For this review, take the finished solid that the model builds, in its own axes (mm). Face numbers are marked on the shaded views. A direction names the side the tool comes from. Coordinates: 2 decimals unless noted, no trailing zeros. Order: outer loops, then holes, each group sorted by start corner. A loop starts at its lowest first (then second) coordinate and runs counter-clockwise, first axis right, second up. Notation, with made-up numbers: (28, 37.5) -> (65, 37.5) arc R37 cw to (65, 73.5) -> close; hole circle Ø8 at (57, 47.25). An arc over 180 degrees is marked (long way). Answer as a JSON object with one key per item and string values. Group by question number.
1) Add section B-B, the plane z = 1.75. Write out the cut boundary in (x, y), then the cut area to 3 significant figures.
2) For pin 1 (4 mm diameter, centred on x = -3, z = 0, fed in from +Y); pin 2 (4 mm diameter, centred on x = -2.5, z = 3, fed in from +Y); pin 3 (6.5 mm diameter, centred on y = -21, z = 4, fed in from +X), all flat-tipped, find the tip position at first contact; note any pin that passes through.
3) Wall thickness on L1, parallel to Y at x = 0.45, z = 5; L2, parallel to Z at x = 2, y = -20.6; L3, parallel to X at y = -10, z = 3.25: over which ranges is each line inside the solid? List them lowest first.
4) Add section A-A, the plane y = -20.6. Write out the cut boundary in (x, z), then the cut area to 3 significant figures.
5) Machinability: for the marked faces 1, 2, 3 and 4, which of the approach directions +Z, -Z, +X, -X, +Y, -Y give a long, thin tool a straight path to every point of the face, cutting with its end or side? Answer none if there is none.
6) Add section C-C, the plane y = -9.15. Write out the cut boundary in (x, z).
7) Draft analysis for pull direction Y (two halves, no side actions). For the marked faces 5, 6 and 7, state which applies: +Y half, -Y half, draft (parallel to the pull), parting line (faces both ways), or undercut.
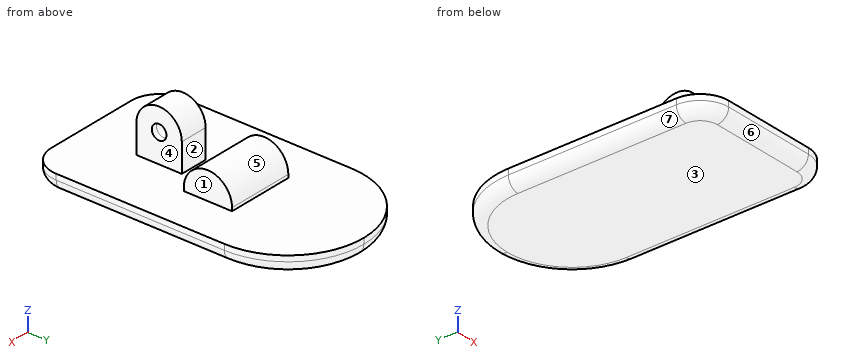
from build123d import *

# Parameters (mm, degrees)
F0_W      = 10.85
F0_H      = 10
F0_W_2    = 2.5
F0_H_2    = 8
F0_W_3    = 7.45
F0_H_3    = 3.2
F0_H_4    = 8.5
F0_W_4    = 5.9
F1_DEPTH  = 3
F2_DEPTH  = 0.563
F3_DEPTH  = 5
F6_DEPTH  = 11.8
F7_DEPTH  = 5
F8_DEPTH  = 25
F9_R      = 2.056128731
F10_DEPTH = 1
F11_R     = 5
F12_R     = 5
F13_R     = 2
F14_DEPTH = 25


with BuildPart() as f1:
    # F0 (on Top) → F1 (new body)
    with BuildSketch(Plane.XY):
        Polygon((-5.9, -16.6), (-13.35, -16.6), (-13.35, -24.6), (-2.5, -24.6), (-2.5, -16.6), align=None)
        with Locations((-7.925, -29.6)):
            Rectangle(F0_W, F0_H)
        with Locations((1.25, -29.6)):
            Rectangle(F0_W_2, F0_H)
        with Locations((-1.25, -29.6)):
            Rectangle(F0_W_2, F0_H)
        with Locations((-1.25, -20.6)):
            Rectangle(F0_W_2, F0_H_2)
        with Locations((1.25, -20.6)):
            Rectangle(F0_W_2, F0_H_2)
        Polygon((13.35, -24.6), (13.35, -16.6), (5.9, -16.6), (2.5, -16.6), (2.5, -24.6), align=None)
        with Locations((7.925, -29.6)):
            Rectangle(F0_W, F0_H)
        Polygon((5.9, -13.4), (0, -13.4), (0, -16.6), (2.5, -16.6), (5.9, -16.6), align=None)
        with Locations((9.625, -15)):
            Rectangle(F0_W_3, F0_H_3)
        Polygon((0, -16.6), (0, -13.4), (-5.9, -13.4), (-5.9, -16.6), (-2.5, -16.6), align=None)
        with Locations((-9.625, -15)):
            Rectangle(F0_W_3, F0_H_3)
        with Locations((-9.625, -9.15)):
            Rectangle(F0_W_3, F0_H_4)
        with Locations((-2.95, -9.15)):
            Rectangle(F0_W_4, F0_H_4)
        with Locations((2.95, -9.15)):
            Rectangle(F0_W_4, F0_H_4)
        with Locations((9.625, -9.15)):
            Rectangle(F0_W_3, F0_H_4)
        with BuildLine():
            Line((13.35, -4.9), (13.35, 0))
            ThreePointArc((13.35, 0), (9.4398755288, 9.4398755288), (0, 13.35))
            Line((0, 13.35), (0, -4.9))
            Line((0, -4.9), (5.9, -4.9))
            Line((5.9, -4.9), (13.35, -4.9))
        make_face()
        with BuildLine():
            Line((0, -4.9), (0, 13.35))
            ThreePointArc((0, 13.35), (-9.4398755288, 9.4398755288), (-13.35, 0))
            Line((-13.35, 0), (-13.35, -4.9))
            Line((-13.35, -4.9), (-5.9, -4.9))
            Line((-5.9, -4.9), (0, -4.9))
        make_face()
    extrude(amount=-F1_DEPTH)

    # F0 (on Top) → F2 (join)
    with BuildSketch(Plane.XY):
        with Locations((-2.95, -9.15)):
            Rectangle(F0_W_4, F0_H_4)
        with Locations((2.95, -9.15)):
            Rectangle(F0_W_4, F0_H_4)
    extrude(amount=F2_DEPTH)

    # F0 (on Top) → F3 (join)
    with BuildSketch(Plane.XY):
        with Locations((1.25, -20.6)):
            Rectangle(F0_W_2, F0_H_2)
        with Locations((-1.25, -20.6)):
            Rectangle(F0_W_2, F0_H_2)
    extrude(amount=F3_DEPTH)

    # F5 (on face) → F6 (join)
    with BuildSketch(Plane.YZ.offset(5.9)):
        with BuildLine():
            Line((-13.4, 0.563), (-4.9, 0.563))
            ThreePointArc((-4.9, 0.563), (-9.15, 4.813), (-13.4, 0.563))
        make_face()
    extrude(amount=-F6_DEPTH)

    # F4 (on face) → F7 (join)
    with BuildSketch(Plane.YZ.offset(2.5)):
        with BuildLine():
            Line((-19.311, 5), (-16.6, 5))
            ThreePointArc((-16.6, 5), (-20.6, 9), (-24.6, 5))
            Line((-24.6, 5), (-21.889, 5))
            ThreePointArc((-21.889, 5), (-20.6, 6.289), (-19.311, 5))
        make_face()
    extrude(amount=-F7_DEPTH)

    # F4 (on face) → F8 (cut)
    with BuildSketch(Plane.YZ.offset(2.5)):
        with BuildLine():
            ThreePointArc((-21.889, 5), (-20.6, 3.711), (-19.311, 5))
            Line((-19.311, 5), (-21.889, 5))
        make_face()
        with BuildLine():
            Line((-21.889, 5), (-19.311, 5))
            ThreePointArc((-19.311, 5), (-20.6, 6.289), (-21.889, 5))
        make_face()
    extrude(amount=-F8_DEPTH, mode=Mode.SUBTRACT)

    # F9 (on face) → F10 (join)
    with BuildSketch(Plane.YZ.offset(2.5)):
        with Locations((-20.6, 5)):
            Circle(F9_R)
    extrude(amount=-F10_DEPTH)

    # F11
    f11_edges = [f1.edges().sort_by_distance(p)[0] for p in [
        (13.35, -34.6, -1.5),
    ]]
    fillet(f11_edges, radius=F11_R)

    # F12
    f12_edges = [f1.edges().sort_by_distance(p)[0] for p in [
        (-13.35, -34.6, -1.5),
    ]]
    fillet(f12_edges, radius=F12_R)

    # F13
    f13_edges = [f1.edges().sort_by_distance(p)[0] for p in [
        (0, -34.6, -3),
    ]]
    fillet(f13_edges, radius=F13_R)

    # F14 (cut): a face of the model
    f14_faces = [f1.faces().sort_by_distance(p)[0] for p in [
        (1.5, -20.6, 5),
    ]]
    extrude(f14_faces, amount=-F14_DEPTH, mode=Mode.SUBTRACT)


solid = f1.part
Output values:
{
 "1": {"outline": "(-5.9, -13.23) -> (5.9, -13.23) -> (5.9, -5.07) -> (-5.9, -5.07) -> close; (-2.5, -24.6) -> (2.5, -24.6) -> (2.5, -16.6) -> (-2.5, -16.6) -> close", "area": "136 mm²"},
 "2": {"pin 1": "stops at y = 13.31", "pin 2": "stops at y = -4.92", "pin 3": "stops at x = 2.5"},
 "3": {"L1": "y = -24.6 to -21.89, -19.31 to -16.6", "L2": "z = -3 to 3.71, 6.29 to 9", "L3": "x = -5.9 to 5.9"},
 "4": {"outline": "(-13.35, -1) arc R2 ccw to (-11.35, -3) -> (11.35, -3) arc R2 ccw to (13.35, -1) -> (13.35, 0) -> (2.5, 0) -> (2.5, 3.71) -> (-2.5, 3.71) -> (-2.5, 0) -> (-13.35, 0) -> close; (-2.5, 6.29) -> (2.5, 6.29) -> (2.5, 9) -> (-2.5, 9) -> close", "area": "110 mm²"},
 "5": {"face 1": "+Z, +X, +Y, -Y", "face 2": "+Z, +X, -X", "face 3": "-Z, +X, -X, +Y, -Y", "face 4": "+Z, +X, -Y"},
 "6": {"outline": "(-13.35, -1) arc R2 ccw to (-11.35, -3) -> (11.35, -3) arc R2 ccw to (13.35, -1) -> (13.35, 0) -> (5.9, 0) -> (5.9, 4.81) -> (-5.9, 4.81) -> (-5.9, 0) -> (-13.35, 0) -> close"},
 "7": {"face 5": "undercut", "face 6": "-Y half", "face 7": "draft"}
}
